Geometry: see drawing. Coordinates: mm, zero at the bounding-box minimum. A direction names the side the tool comes from. Give positions to 0.01 mm unless a question says otherwise; leave off trailing zeros. Write each loop counter-clockwise with the first axis right and the second up, starting at its lowest first coordinate (ties: lowest second). Pieces come first, ordered by that corner, then holes. Notation, with made-up numbers: (51, 30) - (74, 30) arc R32 cw to (74, 65) - close; hole circle Ø3 at (29, 85.5). An arc over 180 degrees is marked (long way). Return JSON: item names as keys, results as strings.
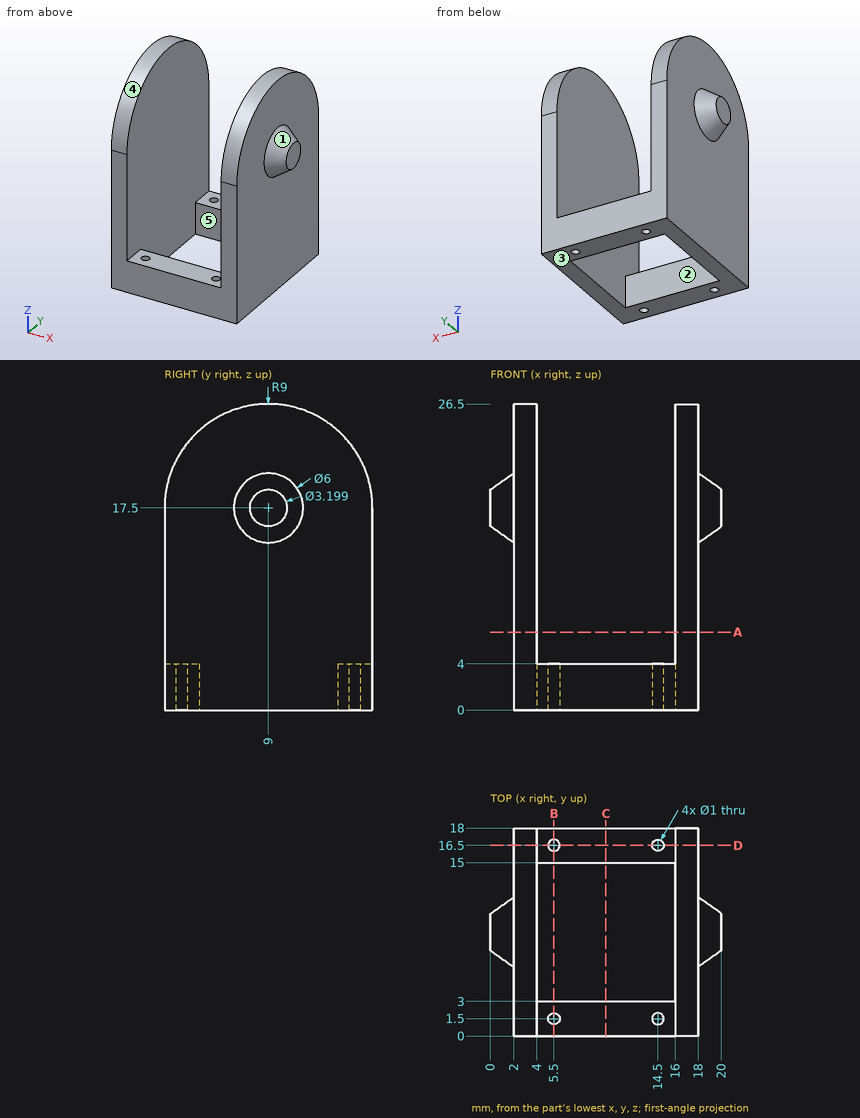
Q1. Section query A-A, the plane z = 6.75. Return the cut outline in (x, y).
Answer key:
{"outline": "(2, 0) - (4, 0) - (4, 18) - (2, 18) - close; (16, 0) - (18, 0) - (18, 18) - (16, 18) - close"}
Q2. Section query B-B, the plane x = 5.5. Return the cut outline in (y, z).
Answer key:
{"outline": "(0, 0) - (1, 0) - (1, 4) - (0, 4) - close; (2, 0) - (3, 0) - (3, 4) - (2, 4) - close; (15, 0) - (16, 0) - (16, 4) - (15, 4) - close; (17, 0) - (18, 0) - (18, 4) - (17, 4) - close"}
Q3. Set-up query: the marked faces 4 and 5. Return all of +Z, -Z, +X, -X, +Y, -Y with unobstructed straight access to the full face (end or side cutting, diameter ignored); none if empty.
Answer key:
{"face 4": "+Z, +X, -X", "face 5": "+Z, -Z"}
Q4. Section query C-C, the plane x = 10. Return the cut outline in (y, z).
Answer key:
{"outline": "(0, 0) - (3, 0) - (3, 4) - (0, 4) - close; (15, 0) - (18, 0) - (18, 4) - (15, 4) - close"}
Q5. Pin query (flat end, axial travel): P1, Ø1, axis at y = 13, z = 9.5, coming from the -X side; P2, Ø3, axis at y = 3.5, z = 21, coming from the +X side; P3, Ø5.5, axis at y = 7.5, z = 12.5, coming from the +X side; P4, Ø8, axis at x = 6, y = 15, coming from the -Z side. Return the tip coordinate at first contact, or that it passes through.
Answer key:
{"P1": "stops at x = 2", "P2": "stops at x = 18", "P3": "stops at x = 18.76", "P4": "stops at z = 0"}
Q6. Material intervals for probe 1 along Y at (x, z) = (5.5, 3.05); probe 2 along X at (y, z) = (1.5, 1); probe 3 along X at (y, z) = (3, 17), sorted ascending. Write a range as [from, to].
Answer key:
{"probe 1": "y = [0, 1], [2, 3], [15, 16], [17, 18]", "probe 2": "x = [2, 5], [6, 14], [15, 18]", "probe 3": "x = [2, 4], [16, 18]"}
Q7. Section query D-D, the plane y = 16.5. Return the cut outline in (x, z) (3 decimals).
Answer key:
{"outline": "(2, 0) - (5, 0) - (5, 4) - (4, 4) - (4, 22.475) - (2, 22.475) - close; (6, 0) - (14, 0) - (14, 4) - (6, 4) - close; (15, 0) - (18, 0) - (18, 22.475) - (16, 22.475) - (16, 4) - (15, 4) - close"}
Q8. Mould query, pull axis X, two halves, no side actions, for the marked faces 1, 2 and 3. Classes: pulls with the +X half, pulls with the -X half, needs draft (parallel to the pull), parting line crosses it, or undercut.
Answer key:
{"face 1": "pulls with the +X half", "face 2": "undercut", "face 3": "needs draft"}
